```python
from build123d import *

# Parameters (mm, degrees)
F0_W     = 50.8
F0_H     = 8.382
F1_DEPTH = 7.62
F3_D     = 6.7564
F3_DEPTH = 23.3426
F3_TIP   = 2.0298273432
F5_DEPTH = 25.4
F6_R     = 5.08


with BuildPart() as f1:
    # F0 (on Front) → F1 (new body)
    with BuildSketch(Plane.XZ):
        Rectangle(F0_W, F0_H)
    extrude(amount=F1_DEPTH)

    # F3
    with Locations(Plane.XZ.offset(7.62)):
        with Locations((-12.2682, 0), (12.2682, 0)):
            Hole(F3_D / 2, depth=F3_DEPTH)
            with Locations((0, 0, -(F3_DEPTH + F3_TIP / 2))):  # 118° drill point
                Cone(0, F3_D / 2, F3_TIP, mode=Mode.SUBTRACT)

    # F4 (on face) → F5 (cut)
    with BuildSketch(Plane.XZ.offset(7.62)):
        with BuildLine():
            Line((6.3864027151, 4.191), (8.9947894332, 0.8348763389))
            ThreePointArc((8.9947894332, 0.8348763389), (12.2692015488, 3.3781998515), (15.5421050298, 0.8329352293))
            Line((15.5421050298, 0.8329352293), (18.1520003825, 4.191))
            Line((18.1520003825, 4.191), (6.3864027151, 4.191))
        make_face()
    extrude(amount=-F5_DEPTH, mode=Mode.SUBTRACT)

    # F6
    f6_edges = [f1.edges().sort_by_distance(p)[0] for p in [
        (8.994789, -3.81, 0.834876),
        (15.542105, -3.81, 0.832935),
    ]]
    fillet(f6_edges, radius=F6_R)


solid = f1.part
```
Geometry check sheet. Reference: the model listing, model coordinates, mm. A direction names the side the tool comes from. Coordinates: 2 decimals unless noted, no trailing zeros. Write each loop counter-clockwise with the first axis right and the second up, starting at its lowest first coordinate (ties: lowest second). Pieces come first, ordered by that corner, then holes. Notation, with made-up numbers: M -24,76.25 L 4,76.25 A18 cw 4,87.25 Z; hole C 66.5,55 d4. An arc over 180 degrees is marked long. One line per item, written item: value. Start each with the question number.
(1) Tool access check on faces 5 (the face through (0, 0, 0)), 6 (the face through (8.562, -3.757, 1.075)). Record the directions out of +Z, -Z, +X, -X, +Y, -Y that give a thin tool (end or side, any length) a straight path to the whole face; none if there is none.
(2) Sectioned sample at C-C, the plane z = 1.25. Enter the section's corners in (x, y).
(3) Release check for a two-part mould opening along Z. For faces 1 (the face through (0, -4, -4.191)), 2 (the face through (-8.893, -3.757, 0.149)), 3 (the face through (22, -4, 4.191)), 4 (the face through (-25.4, -4, 0)) record: released by +Z, released by -Z, zero draft, split by the parting line, or undercut.
(4) Sectioned sample at B-B, the plane z = -0.75. Enter the section's corners in (x, y).
(5) Sectioned sample at D-D, the plane x = 11.5. Enter the section's corners in (y, z).
(6) Sectioned sample at A-A, the plane y = -4.25. Enter the section's corners in (x, z).
(7) Scan lines: line 1 along X through (y, z) = (-4.5, 2.75); line 2 along X through (y, z) = (-2.5, 1.25); line 3 along Z through (x, y) = (-13.5, -1.75). Record each from-to range of solid material in increasing order. Write a range as [from, to].
Filled sheet:
1. face 5: +Z, -Z, +X, -X, +Y
1. face 6: +Z, +Y, -Y
2. outline: M -25.4,-7.62 L -15.41,-7.62 L -15.41,0 L -25.4,0 Z; M -9.13,-7.62 L 8.49,-7.62 L 8.49,0 L -9.13,0 Z; M 16.05,-7.62 L 25.4,-7.62 L 25.4,0 L 16.05,0 Z
3. face 1: released by -Z
3. face 2: undercut
3. face 3: released by +Z
3. face 4: zero draft
4. outline: M -25.4,-7.62 L -15.56,-7.62 L -15.56,0 L -25.4,0 Z; M -8.97,-7.62 L 8.97,-7.62 L 8.97,0 L -8.97,0 Z; M 15.56,-7.62 L 25.4,-7.62 L 25.4,0 L 15.56,0 Z
5. outline: M -7.62,-4.19 L 0,-4.19 L 0,-3.29 L -7.62,-3.29 Z
6. outline: M -25.4,-4.19 L 25.4,-4.19 L 25.4,4.19 L 18.15,4.19 L 16.67,2.29 A5.08 ccw 15.63,-0.33 A3.38 cw 8.91,-0.33 A5.08 ccw 7.86,2.29 L 6.39,4.19 L -25.4,4.19 Z; hole C -12.27,0 d6.76
7. line 1: [-25.4, -14.23], [-10.31, 7.51], [17.03, 25.4]
7. line 2: [-25.4, -15.41], [-9.13, 8.49], [16.05, 25.4]
7. line 3: [-4.19, -3.15], [3.15, 4.19]
